CAD build for the part. Positions are in the model's coordinates, mm. Face numbers are marked on the shaded views. A direction names the side the tool comes from. Give positions to 0.01 mm unless a question says otherwise; leave off trailing zeros. Order: outer loops, then holes, each group sorted by start corner. A loop starts at its lowest first (then second) coordinate and runs counter-clockwise, first axis right, second up.
Item 1: Two-plate mould, pull along X, no slides. Class the marked faces 1, 2 and 3: released by +X, released by -X, zero draft, split by the parting line, or undercut.
Item 2: Wall check: L1, parallel to Y at x = 8.25, z = 5.25; L2, parallel to Z at x = 15.25, y = 13.5. Give the ranges that are in metal, low to high.
Item 3: Band-saw the part on C-C on y = 12.5. Give the cut face in (x, z), plus the area to 3 significant figures.
Item 4: Which spindle directions (+Z, -Z, +X, -X, +Y, -Y) get a long thin tool onto all of the face, cutting with end or side? Do the marked faces 4, 5 and 6. Say none if no direction does.
Item 5: Flat gauge pins, fed straight in: P1, Ø8, axis at y = 7, z = 15.5, coming from the +X side; P2, Ø1, axis at y = 6.5, z = 8, coming from the +X side; P3, Ø3, axis at x = 7, y = 8, coming from the -Z side; P4, Ø8, axis at y = 14.5, z = 22, coming from the +X side. Where does each tip first touch, or does it go through?
Item 6: Band-saw the part on B-B on x = -5.5. Give the cut face in (y, z), plus the area to 3 significant figures.
Item 7: Band-saw the part on A-A on z = 9. Give the cut face in (x, y).
Item 8: Band-saw the part on D-D on y = 2.25. Give the cut face in (x, z).
```python
from build123d import *

# Parameters (mm, degrees)
SKETCH_1_W          = 16
SKETCH_1_H          = 16
SKETCH_1_W_2        = 10
SKETCH_1_H_2        = 10
EXTRUDE_1_DEPTH     = 10
EXTRUDE_2_DEPTH     = 16
EXTRUDE_3_DEPTH     = 5
EXTRUDE_5_DEPTH     = 16
SKETCH_12_W         = 6
SKETCH_12_H         = 3
CUT_EXTRUDE_2_DEPTH = 8
CUT_EXTRUDE_3_DEPTH = 16


with BuildPart() as part:
    # 草图1 → 凸台-拉伸1 (new body)
    with BuildSketch(Plane.XY):
        with Locations((8, 8)):
            Rectangle(SKETCH_1_W, SKETCH_1_H)
        with Locations((8, 8)):
            Rectangle(SKETCH_1_W_2, SKETCH_1_H_2, mode=Mode.SUBTRACT)
    extrude(amount=EXTRUDE_1_DEPTH)

    # 草图2 → 凸台-拉伸2 (add)
    with BuildSketch(Plane.XZ):
        Polygon((0, 10), (0, 26), (16, 10), align=None)
    extrude(amount=-EXTRUDE_2_DEPTH)

    # 草图6 → 凸台-拉伸3 (add)
    with BuildSketch(Plane(origin=(13, 0, 13), x_dir=(0.7071067811865475, 0, -0.7071067811865477), z_dir=(0.7071067811865477, 0, 0.7071067811865475))):
        with BuildLine():
            ThreePointArc((-7.071067812, 16), (-15.071067812, 8), (-7.071067812, 0))
            Line((-7.071067812, 0), (-7.071067812, 16))
        make_face()
        with BuildLine():
            Line((-7.071067812, 16), (-7.071067812, 0))
            ThreePointArc((-7.071067812, 0), (-1.414213562, 2.343145751), (0.928932188, 8))
            ThreePointArc((0.928932188, 8), (-1.414213562, 13.656854249), (-7.071067812, 16))
        make_face()
    extrude(amount=EXTRUDE_3_DEPTH)

    # 草图10 → 凸台-拉伸5 (add)
    with BuildSketch(Plane(origin=(0, 16, 0), x_dir=(1, 0, 0), z_dir=(0, 1, 0))):
        Polygon((0, -26), (-3.535533906, -29.535533906), (-7.778174593, -25.292893219), (0, -17.514718626), align=None)
    extrude(amount=-EXTRUDE_5_DEPTH)

    # 草图12 → 切除-拉伸2 (cut)
    with BuildSketch(Plane(origin=(-16.535533906, 0, 16.535533906), x_dir=(0.7071067811865475, 0, 0.7071067811865477), z_dir=(-0.7071067811865477, 0, 0.7071067811865475))):
        with Locations((15.384776311, 8)):
            Rectangle(SKETCH_12_W, SKETCH_12_H)
    extrude(amount=-CUT_EXTRUDE_2_DEPTH, mode=Mode.SUBTRACT)

    # 草图13 → 切除-拉伸3 (cut)
    with BuildSketch(Plane(origin=(0, 16, 0), x_dir=(1, 0, 0), z_dir=(0, 1, 0))):
        with BuildLine():
            ThreePointArc((-4.596194078, -24.939339828), (-4.596194078, -26.353553391), (-3.181980515, -26.353553391))
            Line((-3.181980515, -26.353553391), (-4.596194078, -24.939339828))
        make_face()
        with BuildLine():
            Line((-4.596194078, -24.939339828), (-3.181980515, -26.353553391))
            ThreePointArc((-3.181980515, -26.353553391), (-2.965207764, -26.029130042), (-2.889087297, -25.646446609))
            ThreePointArc((-2.889087297, -25.646446609), (-3.506403864, -24.722567077), (-4.596194078, -24.939339828))
        make_face()
    extrude(amount=-CUT_EXTRUDE_3_DEPTH, mode=Mode.SUBTRACT)


solid = part.part
```
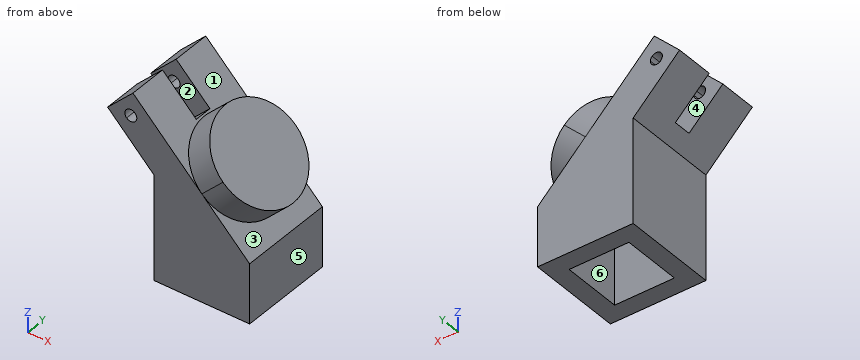
The answers:
1. face 1: undercut
1. face 2: zero draft
1. face 3: released by +X
2. L1: y = 0 to 3, 13 to 16
2. L2: z = 0 to 10.75, 17.03 to 17.82
3. outline: (-7.78, 25.29) - (0, 17.51) - (0, 0) - (3, 0) - (3, 10) - (13, 10) - (13, 0) - (16, 0) - (16, 10) - (12.68, 13.32) - (16.21, 16.86) - (6.86, 26.21) - (3.32, 22.68) - (-3.54, 29.54) - close; hole circle Ø2 at (-3.89, 25.65)
3. area: 299 mm2
4. face 4: +Z, -X
4. face 5: -Z, +X, +Y, -Y
4. face 6: -Z
5. P1: stops at x = 17.19
5. P2: stops at x = 16
5. P3: stops at z = 10
5. P4: stops at x = 15.06
6. outline: (0, 23.01) - (6.5, 23.01) - (6.5, 27.57) - (0, 27.57) - close; (9.5, 23.01) - (16, 23.01) - (16, 27.57) - (9.5, 27.57) - close
6. area: 59.2 mm2
7. outline: (0, 0) - (16, 0) - (16, 16) - (0, 16) - close; hole (3, 3) - (13, 3) - (13, 13) - (3, 13) - close
8. outline: (-7.78, 25.29) - (0, 17.51) - (0, 0) - (16, 0) - (16, 10) - (11.93, 14.07) - (15.47, 17.6) - (7.6, 25.47) - (4.07, 21.93) - (-3.54, 29.54) - close; hole circle Ø2 at (-3.89, 25.65)
